Here's how the part is built. I have some questions about the finished solid (model axes, mm). A direction names the side the tool comes from. Give positions to 0.01 mm unless a question says otherwise; leave off trailing zeros. Order: outer loops, then holes, each group sorted by start corner. A loop starts at its lowest first (then second) coordinate and runs counter-clockwise, first axis right, second up.
Autodesk Inventor part; units mm, degrees
ref_plane "YZ Plane" through (0, 0, 0) normal (1, 0, 0) x (0, 1, 0)
ref_plane "XZ Plane" through (0, 0, 0) normal (0, 1, 0) x (-1, 0, 0)
ref_plane "XY Plane" through (0, 0, 0) normal (0, 0, 1) x (1, 0, 0)
sketch "スケッチ1" plane through (0, 0, 0) normal (0, 0, 1) x (1, 0, 0)
  line L0 (14.5, 10) -> (-14.5, 10)
  line L1 (-14.5, 10) -> (-14.5, -10)
  line L2 (-14.5, -10) -> (14.5, -10)
  line L3 (14.5, -10) -> (14.5, 10)
  line L4 (14.5, 10) -> (-14.5, -10) construction
  line L5 (-14.5, 10) -> (14.5, -10) construction
  point P0 (0, 0)
  dimension "d0" = 29
  dimension "d1" = 20
extrude "押し出し1" add sketch "スケッチ1" along normal blind 8.1
sketch "スケッチ2" plane through (0, 0, 8.1) normal (0, 0, 1) x (1, 0, 0)
  circle A0 centre (-5, 7.5) radius 1.5
  circle A1 centre (5, 7.5) radius 1.5
  circle A2 centre (5, -7.5) radius 1.5
  circle A3 centre (-5, -7.5) radius 1.5
  point P0 (0, 0)
  dimension "d4" = 3
  dimension "d5" = 3
  dimension "d6" = 3
  dimension "d7" = 3
extrude "押し出し2" cut sketch "スケッチ2" against normal blind 4
thread "ねじ1"
thread "ねじ2"
thread "ねじ3"
thread "ねじ4"
sketch "スケッチ3" plane through (0, 0, 0) normal (0, 0, -1) x (-1, 0, 0)
  line L0 (-14.5, -10) -> (-14.5, 10)
  line L1 (14.5, -4.5) -> (-14.5, -4.5)
  line L2 (-14.5, -4.5) -> (-14.5, 4.5)
  line L3 (-14.5, 4.5) -> (14.5, 4.5)
  line L4 (14.5, 4.5) -> (14.5, -4.5)
  line L5 (14.5, -4.5) -> (-14.5, 4.5) construction
  line L6 (-14.5, -4.5) -> (14.5, 4.5) construction
  point P0 (0, 0)
  dimension "d18" = 9
extrude "押し出し3" cut sketch "スケッチ3" against normal blind 5.1
chamfer "面取り1" distance 0.5 angle 45 6 edges at (0, 10, 8.1) (0, -10, 8.1) (0, -10, 0) (0, 10, 0) (0, -4.5, 0) (0, 4.5, 0)
properties part number "slider" material "ステンレス鋼"
Q1. If we section it at C-C on z = 7: List the corners of the cut face in (x, y) for me, plus the area to 3 significant figures.
Filled sheet:
outline: (-14.5, -10) - (14.5, -10) - (14.5, 10) - (-14.5, 10) - close; hole circle Ø3 at (-5, -7.5); hole circle Ø3 at (-5, 7.5); hole circle Ø3 at (5, -7.5); hole circle Ø3 at (5, 7.5)
area: 552 mm2
Q2. I need wall thicknesses on L1, parallel to Y at x = -5, z = 7; L2, parallel to X at y = 6.5, z = 6.75; L3, parallel to Y at x = -5, z = 3.75. Which ranges of each line are inside material? Lowest first, please.
Filled sheet:
L1: y = -10 to -9, -6 to 6, 9 to 10
L2: x = -14.5 to -6.12, -3.88 to 3.88, 6.12 to 14.5
L3: y = -10 to -4.5, 4.5 to 10
Q3. I'm going to push flat-ended pins straight in: P1, Ø0.9, axis at x = -4.5, y = -7.5, coming from the +Z side; P2, Ø4.5, axis at x = -0.5, y = -2, coming from the -Z side. Where does each tip first touch, or does it pass through?
Filled sheet:
P1: stops at z = 4.1
P2: stops at z = 5.1
Q4. If we section it at B-B on x = 9.75: List the corners of the cut face in (y, z) for me.
Filled sheet:
outline: (-10, 0.5) - (-9.5, 0) - (-5, 0) - (-4.5, 0.5) - (-4.5, 5.1) - (4.5, 5.1) - (4.5, 0.5) - (5, 0) - (9.5, 0) - (10, 0.5) - (10, 7.6) - (9.5, 8.1) - (-9.5, 8.1) - (-10, 7.6) - close
Q5. If we section it at A-A on z = 4.5: List the corners of the cut face in (x, y) for me.
Filled sheet:
outline: (-14.5, -10) - (14.5, -10) - (14.5, -4.5) - (-14.5, -4.5) - close; (-14.5, 4.5) - (14.5, 4.5) - (14.5, 10) - (-14.5, 10) - close; hole circle Ø3 at (-5, -7.5); hole circle Ø3 at (-5, 7.5); hole circle Ø3 at (5, -7.5); hole circle Ø3 at (5, 7.5)
Q6. Thinking about a two-plate mould opening in X: for faces 1 (the face through (14.5, 0, 6)), 2 (the face through (-14.5, 0, 6)), 3 (the face through (0, 7, 0)), 4 (the face through (5.69, 6.17, 6.13)), which applies, released by +X, released by -X, zero draft, split by the parting line, or undercut?
Filled sheet:
face 1: released by +X
face 2: released by -X
face 3: zero draft
face 4: undercut
Q7. If we section it at D-D on z = 1: List the corners of the cut face in (x, y) for me, plus the area to 3 significant figures.
Filled sheet:
outline: (-14.5, -10) - (14.5, -10) - (14.5, -4.5) - (-14.5, -4.5) - close; (-14.5, 4.5) - (14.5, 4.5) - (14.5, 10) - (-14.5, 10) - close
area: 319 mm2
Q8. For faces 5 (the face through (5, -7, 4.1)), 6 (the face through (0, 10, 4)), 7 (the face through (0, 4.5, 3)), which set-ups out of +Z, -Z, +X, -X, +Y, -Y let a thin tool reach every point of the face, with its end or its side?
Filled sheet:
face 5: +Z
face 6: +Z, -Z, +X, -X, +Y
face 7: -Z, +X, -X
